For this review, take the finished solid that the model builds, in its own axes (mm). A direction names the side the tool comes from. Round coordinates to 2 decimals unless told otherwise and drop trailing zeros. Order: outer loops, then holes, each group sorted by start corner. A loop starts at its lowest first (then second) coordinate and runs counter-clockwise, first axis right, second up. Notation, with made-up numbers: M 29,-30.5 L 48,-30.5 A26 cw 48,-8.5 Z; hole C -30.75,-33.75 d5. An arc over 180 degrees is marked long. Answer in a Markdown table with one row per item. Add a question column.
Autodesk Inventor part; units mm, degrees
ref_plane "YZ Plane" through (0, 0, 0) normal (1, 0, 0) x (0, 1, 0)
ref_plane "XZ Plane" through (0, 0, 0) normal (0, 1, 0) x (-1, 0, 0)
ref_plane "XY Plane" through (0, 0, 0) normal (0, 0, 1) x (1, 0, 0)
sketch "Sketch1" plane through (0, 0, 0) normal (0, 0, 1) x (1, 0, 0)
  line L0 (0, 0) -> (19.05, 0)
  line L1 (19.05, 0) -> (19.05, 19.05)
  line L2 (19.05, 19.05) -> (18.2563, 19.05)
  line L3 (18.2563, 19.05) -> (18.2563, 0.7938)
  line L4 (18.2563, 0.7938) -> (0, 0.7937)
  line L5 (0, 0.7937) -> (0, 0)
  dimension "d0" = 19.05
  dimension "d1" = 19.05
  dimension "d2" = 0.7937
extrude "Extrusion1" add sketch "Sketch1" along normal blind 260.35
sketch "Sketch2" plane through (0, 0, 260.35) normal (0, 0, 1) x (1, 0, 0)
  line L0 (0, 0) -> (19.05, 0)
  line L1 (19.05, 0) -> (19.05, 19.05)
  line L2 (19.05, 19.05) -> (18.2563, 19.05)
  line L3 (18.2563, 19.05) -> (18.2563, 0.7938)
  line L4 (18.2563, 0.7938) -> (18.2563, 0)
extrude "Extrusion2" cut sketch "Sketch2" against normal blind 3.175
sketch "Sketch3" plane through (18.2563, 0, 259.5563) normal (0, 0, 1) x (1, 0, 0)
  line L0 (-18.2563, 0) -> (0, 0)
  line L1 (0, 0) -> (0, 19.05)
  line L2 (0, 19.05) -> (-18.2563, 19.05)
  line L3 (-18.2563, 19.05) -> (-18.2563, 0)
edge flange "Flange1" height 19.05 angle 90 thickness 0.7937 bend radius 0.635 thickness toward (0, 0, 1) relief straight relief width 0.7937 relief depth 0.3969 edges at (9.1281, 0.7938, 260.35) wall of the first edge with corners at (0, 0, 259.5563) (18.2563, 0, 259.5563) (18.2562, 19.05, 259.5563) (0, 19.05, 259.5563)
bend "Bend1"
corner "Corner1"
sketch "Sketch4" plane through (0, 19.05, 260.35) normal (0, 0, 1) x (1, 0, 0)
  line L0 (0, -17.6213) -> (18.2563, -17.6213)
  line L1 (0, 0) -> (18.2563, 0)
  circle A0 centre (5.1594, -8.8106) radius 1.5875
  circle A1 centre (13.0969, -8.8106) radius 1.5875
  line L2 (5.1594, -8.8106) -> (13.0969, -8.8106) construction
  line L3 (9.1281, 0) -> (9.1281, -17.6213) construction
  point P0 (0, -19.05)
  point P1 (9.1281, -8.8106)
  dimension "d21" = 3.175
  dimension "d22" = 7.9375
extrude "Extrusion3" cut sketch "Sketch4" against normal through all
mirror "Mirror1" about plane through (13.8989, 5.1511, 0) normal (0, 0, -1)
equation "\"d7\" = BendReliefWidth"
equation "\"d8\" = BendReliefDepth"
equation "\"d9\" = MinimumRemnant"
equation "\"d10\" = BendRadius"
equation "\"d14\" = CornerReliefSize"
equation "\"d15\" = GapSize"
equation "\"d16\" = JacobiRadiusSize"
equation "\"BendRadius\" = Thickness"
equation "\"BendReliefWidth\" = Thickness"
equation "\"BendReliefDepth\" = 0.5 * Thickness"
equation "\"CornerReliefSize\" = 4 * Thickness"
equation "\"MinimumRemnant\" = 2 * Thickness"
equation "\"TransitionRadius\" = BendRadius"
equation "\"JacobiRadiusSize\" = Thickness"
equation "\"GapSize\" = Thickness"
properties part number "Climber Connector Bar" material "Aluminum 6061"
1. Clearance check with flat-ended pins moving along their axes: pin 1 Ø1.1 at (y, z) = (10, 259.5) entering from +X; pin 2 Ø9 at (x, z) = (12, -71.5) entering from +Y; pin 3 Ø3.5 at (x, y) = (5.16, 10.24) entering from -Z; pin 4 Ø1.9 at (x, y) = (5.16, 10.24) entering from -Z. State where each tip first meets the part, or that it passes through.
2. Consider section B-B on z = 99. Write out the cut boundary in (x, y), plus the area to 3 significant figures.
3. The part is to be moulded in two halves that separate along Z. For faces 4 (the flat face through (9, 10, 259.556)), 5 (the flat face through (19.05, 9, -4)), 6 (the flat face through (9, 10, -260.35)), say which applies: pulls with the +Z half, pulls with the -Z half, needs draft (parallel to the pull), parting line crosses it, or undercut.
4. Consider section A-A on y = 5.75. Write out the cut boundary in (x, z) (3 decimals), plus the area to 3 significant figures.
5. For faces 1 (the flat face through (9, 10, -259.556)), 2 (the flat face through (9, 10, 260.35)), 3 (the flat face through (18.256, 10, -4)), list the 3-axis set-ups (+Z, -Z, +X, -X, +Y, -Y) from which the entire face can be reached by the end or side of a thin tool; tool diameter is ignored.
6. To check wall thickness, follow probe 1 along Z at (x, y) = (7, 1.5); probe 2 along X at (y, z) = (9.5, 8.5); probe 3 along Y at (x, z) = (8.75, 35). State the ranges of each line that lie inside material, in increasing order. Write a range as [from, to].
Solved:
| question | item | result |
|---|---|---|
| 1 | pin 1 | stops at x = 18.26 |
| 1 | pin 2 | stops at y = 0.79 |
| 1 | pin 3 | stops at z = -260.35 |
| 1 | pin 4 | passes through |
| 2 | outline | M 0,0 L 19.05,0 L 19.05,19.05 L 18.26,19.05 L 18.26,0.79 L 0,0.79 Z |
| 2 | area | 29.6 mm^2 |
| 3 | face 4 | undercut |
| 3 | face 5 | needs draft |
| 3 | face 6 | pulls with the -Z half |
| 4 | outline | M 0,-260.35 L 18.256,-260.35 L 18.256,-259.556 L 0,-259.556 Z; M 0,259.556 L 18.256,259.556 L 18.256,260.35 L 0,260.35 Z; M 18.256,-257.175 L 19.05,-257.175 L 19.05,257.175 L 18.256,257.175 Z |
| 4 | area | 437 mm^2 |
| 5 | face 1 | +X, -X, +Y |
| 5 | face 2 | +Z, +X, -X, +Y, -Y |
| 5 | face 3 | -X, +Y |
| 6 | probe 1 | z = [-260.35, -259.56], [259.56, 260.35] |
| 6 | probe 2 | x = [18.26, 19.05] |
| 6 | probe 3 | y = [0, 0.79] |
